Drawing for the job (mm, zero at the part's lowest x, y, z). A direction names the side the tool comes from. Coordinates: 2 decimals unless noted, no trailing zeros. Loops run counter-clockwise (first coordinate to the right, second up) from the corner with the lowest first, then second, coordinate; pieces in that order, holes last. Notation, with made-up numbers: (89, -14.5) - (120, -14.5) arc R15 cw to (120, 3.5) - close; hole circle Ø5 at (2.5, 2.25). An arc over 180 degrees is marked (long way). One line per item, written item: value.
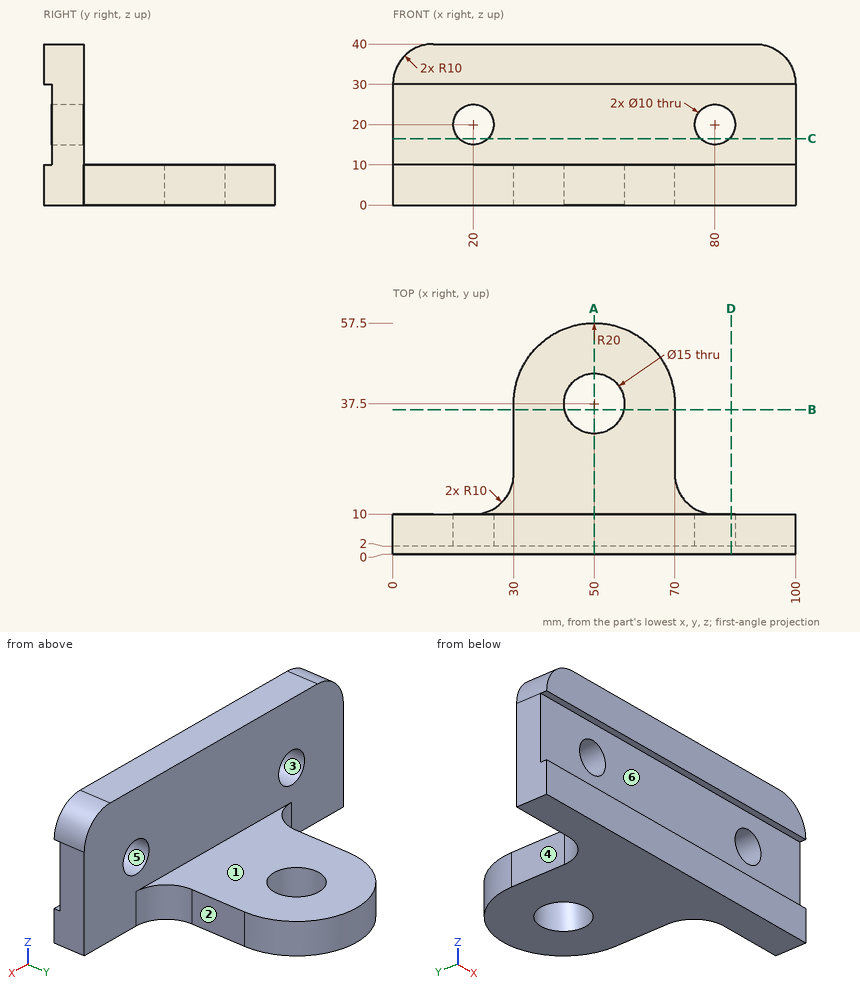
Item 1: Cut at B-B, the plane y = 36. Write the cut outline in (x, z), then the cut area to 3 significant figures.
Check result:
outline: (30, 0) - (42.65, 0) - (42.65, 10) - (30, 10) - close; (57.35, 0) - (70, 0) - (70, 10) - (57.35, 10) - close
area: 253 mm^2
Item 2: Cut at A-A, the plane x = 50. Write the cut outline in (y, z).
Check result:
outline: (0, 0) - (30, 0) - (30, 10) - (10, 10) - (10, 40) - (0, 40) - (0, 30) - (2, 30) - (2, 10) - (0, 10) - close; (45, 0) - (57.5, 0) - (57.5, 10) - (45, 10) - close
Item 3: Probe probe 1 along X at (y, z) = (5, 20); probe 2 along Y at (x, z) = (50, 4); probe 3 along Z at (x, y) = (80, 6). List the from-to ranges inside material, lowest first. Write a range as from..to.
Check result:
probe 1: x = 0..15, 25..75, 85..100
probe 2: y = 0..30, 45..57.5
probe 3: z = 0..15, 25..40
Item 4: Cut at C-C, the plane z = 16.5. Write the cut outline in (x, y).
Check result:
outline: (0, 2) - (16.43, 2) - (16.43, 10) - (0, 10) - close; (23.57, 2) - (76.43, 2) - (76.43, 10) - (23.57, 10) - close; (83.57, 2) - (100, 2) - (100, 10) - (83.57, 10) - close
Item 5: Tool access for the marked faces 4, 5 and 6: list every direction of +Z, -Z, +X, -X, +Y, -Y with a clear straight run to the whole face (end or side of a thin tool).
Check result:
face 4: +Z, -Z, -X, +Y
face 5: +Y, -Y
face 6: +X, -X, -Y
Item 6: Cut at D-D, the plane x = 84. Write the cut outline in (y, z), then the cut area to 3 significant figures.
Check result:
outline: (0, 0) - (10, 0) - (10, 17) - (2, 17) - (2, 10) - (0, 10) - close; (0, 30) - (2, 30) - (2, 23) - (10, 23) - (10, 40) - (0, 40) - close
area: 312 mm^2
Item 7: Drop flat-ended pins along their axis: P1, Ø8, axis at y = 32, z = 6, coming from the -X side; P2, Ø13, axis at x = 20, z = 20, coming from the +Y side; P3, Ø24, axis at x = 55.5, y = 26, coming from the +Z side. Give the stop position or say it passes through.
Check result:
P1: stops at x = 30
P2: stops at y = 10
P3: stops at z = 10
Item 8: Pull direction Z, two halves, no side cores. Call the marked faces 1, 2 and 3: released by +Z, released by -Z, zero draft, split by the parting line, or undercut.
Check result:
face 1: released by +Z
face 2: zero draft
face 3: undercut
